from build123d import *

# Parameters (mm, degrees)
SKETCH1_W           = 24
SKETCH1_H           = 21
BOSS_EXTRUDE1_DEPTH = 2
SKETCH2_W           = 22
SKETCH2_H           = 19
BOSS_EXTRUDE2_DEPTH = 13.5
SKETCH3_W           = 1.2
SKETCH3_H           = 19
BOSS_EXTRUDE3_DEPTH = 6.8
SKETCH4_W           = 4.5
SKETCH4_H           = 0.9
BOSS_EXTRUDE4_DEPTH = 6.8


with BuildPart() as part:
    # Sketch1 → Boss-Extrude1 (new body)
    with BuildSketch(Plane(origin=(0, 0, 0), x_dir=(1, 0, 0), z_dir=(0, 1, 0))):
        Rectangle(SKETCH1_W, SKETCH1_H)
    extrude(amount=BOSS_EXTRUDE1_DEPTH)

    # Sketch2 → Boss-Extrude2 (add)
    with BuildSketch(Plane(origin=(0, 2, 0), x_dir=(1, 0, 0), z_dir=(0, 1, 0))):
        Rectangle(SKETCH2_W, SKETCH2_H)
    extrude(amount=BOSS_EXTRUDE2_DEPTH)

    # Sketch3 → Boss-Extrude3 (add)
    with BuildSketch(Plane(origin=(0, 15.5, 0), x_dir=(1, 0, 0), z_dir=(0, 1, 0))):
        Rectangle(SKETCH3_W, SKETCH3_H)
    extrude(amount=BOSS_EXTRUDE3_DEPTH)

    # Sketch4 → Boss-Extrude4 (add)
    with BuildSketch(Plane(origin=(0, 15.5, 0), x_dir=(1, 0, 0), z_dir=(0, 1, 0))):
        with Locations((-5.25, 7.1)):
            Rectangle(SKETCH4_W, SKETCH4_H)
        with Locations((-5.25, 0)):
            Rectangle(SKETCH4_W, SKETCH4_H)
        with Locations((5.25, 7.1)):
            Rectangle(SKETCH4_W, SKETCH4_H)
        with Locations((5.25, 0)):
            Rectangle(SKETCH4_W, SKETCH4_H)
    extrude(amount=BOSS_EXTRUDE4_DEPTH)


solid = part.part
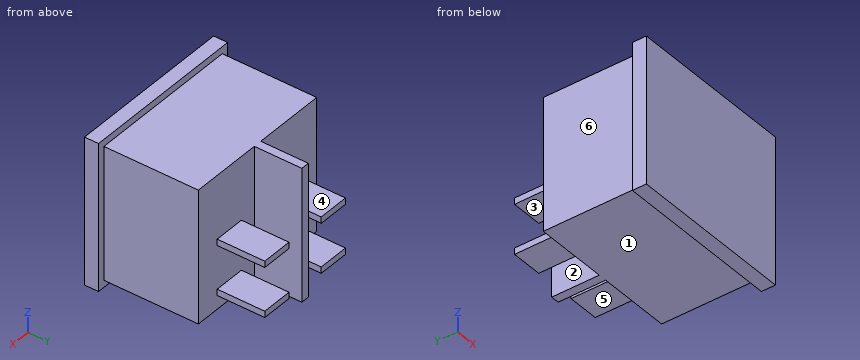
Build history of the part. All positions in model axes, mm. Face numbers are marked on the shaded views. A direction names the side the tool comes from. Round coordinates to 2 decimals unless told otherwise and drop trailing zeros. Loops run counter-clockwise (first coordinate to the right, second up) from the corner with the lowest first, then second, coordinate; pieces in that order, holes last. Notation, with made-up numbers: (44, 37.25) -> (49, 37.25) arc R20 ccw to (49, 49.25) -> close; hole circle Ø5 at (-38.5, 6.5). An arc over 180 degrees is marked (long way). Use CSV: the item, a comma, the result in double quotes. Start each with the question number.
Q1. Mould opens along Z. For the marked faces 1, 2 and 3 say: +Z half, -Z half, draft (parallel to the pull), parting line (faces both ways), or undercut.
Q2. Saw through at B-B on x = 9.75. Give the cut face in (y, z).
Q3. Saw through at A-A on y = 17.75. Give the cut face in (x, z), and give its area (3 significant figures).
Q4. Saw through at C-C on z = -2. Give the cut face in (x, y).
Q5. Drill centre lines: L1, parallel to Z at x = -5.5, y = 20.25; L2, parallel to Y at x = -7, z = 8.5; L3, parallel to X at y = 18, z = 6.75. Where is each one in solid material? Low to high.
Q6. Which spindle directions (+Z, -Z, +X, -X, +Y, -Y) get a long thin tool onto all of the face, cutting with end or side? Do the marked faces 4, 5 and 6. Say none if no direction does.
Q7. Flat gauge pins, fed straight in: pin 1 Ø1.3 at (x, y) = (5.5, 18.5) entering from -Z; pin 2 Ø3 at (y, z) = (5, 2) entering from -X; pin 3 Ø0.5 at (y, z) = (17.5, -7) entering from -X; pin 4 Ø10 at (y, z) = (4, 4.5) entering from +X. Where does each tip first touch, or does it go through?
Q8. Saw through at D-D on x = -6.25. Give the cut face in (y, z), and give its area (3 significant figures).
Solutions:
1,face 1,"-Z half"
1,face 2,"draft"
1,face 3,"undercut"
2,outline,"(0, -10.5) -> (2, -10.5) -> (2, -9.5) -> (15.5, -9.5) -> (15.5, 9.5) -> (2, 9.5) -> (2, 10.5) -> (0, 10.5) -> close"
3,outline,"(-7.5, -7.55) -> (-3, -7.55) -> (-3, -6.65) -> (-7.5, -6.65) -> close; (-7.5, -0.45) -> (-3, -0.45) -> (-3, 0.45) -> (-7.5, 0.45) -> close; (-0.6, -9.5) -> (0.6, -9.5) -> (0.6, 9.5) -> (-0.6, 9.5) -> close; (3, -7.55) -> (7.5, -7.55) -> (7.5, -6.65) -> (3, -6.65) -> close; (3, -0.45) -> (7.5, -0.45) -> (7.5, 0.45) -> (3, 0.45) -> close"
3,area,"39.0 mm^2"
4,outline,"(-12, 0) -> (12, 0) -> (12, 2) -> (11, 2) -> (11, 15.5) -> (0.6, 15.5) -> (0.6, 22.3) -> (-0.6, 22.3) -> (-0.6, 15.5) -> (-11, 15.5) -> (-11, 2) -> (-12, 2) -> close"
5,L1,"z = -7.55 to -6.65, -0.45 to 0.45"
5,L2,"y = 0 to 15.5"
5,L3,"x = -0.6 to 0.6"
6,face 4,"+Z, -X, +Y"
6,face 5,"-Z, +X, +Y"
6,face 6,"+Z, -Z, -X, +Y"
7,pin 1,"stops at z = -7.55"
7,pin 2,"stops at x = -11"
7,pin 3,"stops at x = -7.5"
7,pin 4,"stops at x = 12"
8,outline,"(0, -10.5) -> (2, -10.5) -> (2, -9.5) -> (15.5, -9.5) -> (15.5, -7.55) -> (22.3, -7.55) -> (22.3, -6.65) -> (15.5, -6.65) -> (15.5, -0.45) -> (22.3, -0.45) -> (22.3, 0.45) -> (15.5, 0.45) -> (15.5, 9.5) -> (2, 9.5) -> (2, 10.5) -> (0, 10.5) -> close"
8,area,"311 mm^2"
